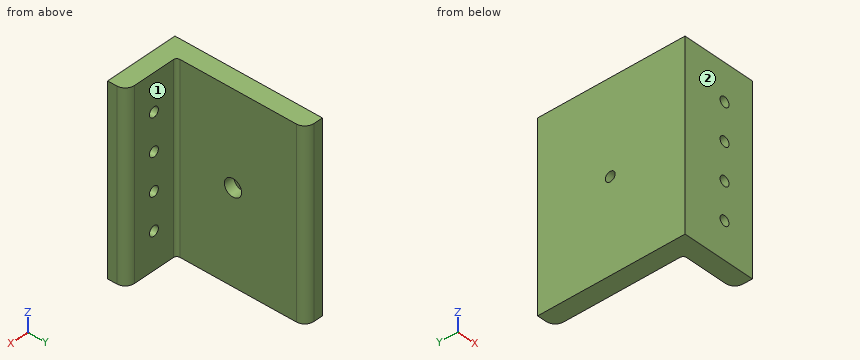
from build123d import *

# Parameters (mm, degrees)
L_ANGLE_L8X4X1_1_DEPTH                   = 254
F_1_2_CLEARANCE_HOLE1_D                  = 13.49248
CBORE_FOR_M12_HEX_HEAD_BOLT1_D           = 13.5
CBORE_FOR_M12_HEX_HEAD_BOLT1_CBORE_D     = 23.78
CBORE_FOR_M12_HEX_HEAD_BOLT1_CBORE_DEPTH = 14.3


with BuildPart() as part:
    # Sketch114 → L angle L8X4X1(1) (new body)
    with BuildSketch(Plane(origin=(390.937425431, -221.174980879, -159.063896304), x_dir=(1, 0, 0), z_dir=(0, 0, 1))):
        with BuildLine():
            Line((0, 0), (0, 203.2))
            Line((0, 203.2), (12.70508, 203.2))
            ThreePointArc((12.70508, 203.2), (21.681744019, 199.481744019), (25.4, 190.50508))
            Line((25.4, 190.50508), (25.4, 30.1625))
            ThreePointArc((25.4, 30.1625), (26.794903955, 26.794903955), (30.1625, 25.4))
            Line((30.1625, 25.4), (88.90508, 25.4))
            ThreePointArc((88.90508, 25.4), (97.881744019, 21.681744019), (101.6, 12.70508))
            Line((101.6, 12.70508), (101.6, 0))
            Line((101.6, 0), (0, 0))
        make_face()
    extrude(amount=L_ANGLE_L8X4X1_1_DEPTH)

    # 1/2 Clearance Hole1 (through all)
    with Locations(Plane(origin=(0, -195.774980879, 0), x_dir=(1, 0, 0), z_dir=(0, 1, 0))):
        with Locations((450.471215431, -44.136103696), (450.471215431, 108.263896304), (450.471215431, 57.463896304), (450.471215431, 6.663896304)):
            Hole(F_1_2_CLEARANCE_HOLE1_D / 2)

    # CBORE for M12 Hex Head Bolt1 (through all)
    with Locations(Plane(origin=(416.337425431, 0, 0), x_dir=(0, 0, -1), z_dir=(1, 0, 0))):
        with Locations((32.063896304, -118.000180879)):
            CounterBoreHole(CBORE_FOR_M12_HEX_HEAD_BOLT1_D / 2, CBORE_FOR_M12_HEX_HEAD_BOLT1_CBORE_D / 2, CBORE_FOR_M12_HEX_HEAD_BOLT1_CBORE_DEPTH)


solid = part.part
Geometry: final body of the model. Coordinates: model frame, mm. Face numbers are marked on the shaded views. A direction names the side the tool comes from. Coordinates: 2 decimals unless noted, no trailing zeros. Order: outer loops, then holes, each group sorted by start corner. A loop starts at its lowest first (then second) coordinate and runs counter-clockwise, first axis right, second up.
(1) First-contact query: pin 1 (12 mm diameter, centred on y = -118.5, z = -29, fed in from +X); pin 2 (8 mm diameter, centred on x = 478.5, z = -68, fed in from +Y) (3 decimals); pin 3 (12 mm diameter, centred on x = 450.47, z = -108.26, fed in from +Y); pin 4 (8 mm diameter, centred on y = -137, z = 38, fed in from +X). Flat tips, straight axial feed; report the tip coordinate or a pass-through.
(2) Section query D-D (z = 12). Return the cut outline in (x, y) (1 decimal).
(3) Section query C-C (y = -121.5). Return the cut outline in (x, z).
(4) Section query B-B (z = -32.5). Return the cut outline in (x, y) (1 decimal).
(5) Material intervals for probe 1 along Z at (x, y) = (414, -118); probe 2 along X at (y, z) = (-131, 40); probe 3 along Y at (x, z) = (471, -53), sorted ascending.
(6) Section query A-A (x = 452.5). Return the cut outline in (y, z), plus the area to 3 significant figures.
(7) Access query for the marked faces 1 and 2. Directions: +Z, -Z, +X, -X, +Y, -Y. A direction counts if a zero-diameter tool reaches every point of the face in a straight line with its end or side. Return the directions, or none.
Solution:
1. pin 1: stops at x = 402.04
1. pin 2: stops at y = -195.775
1. pin 3: passes through
1. pin 4: stops at x = 416.34
2. outline: (390.9, -221.2) - (492.5, -221.2) - (492.5, -208.5) arc R12.7 ccw to (479.8, -195.8) - (421.1, -195.8) arc R4.8 cw to (416.3, -191) - (416.3, -30.7) arc R12.7 ccw to (403.6, -18) - (390.9, -18) - close
3. outline: (390.94, -159.06) - (416.34, -159.06) - (416.34, -43.43) - (402.04, -43.43) - (402.04, -37.84) - (390.94, -37.84) - close; (390.94, -26.29) - (402.04, -26.29) - (402.04, -20.7) - (416.34, -20.7) - (416.34, 94.94) - (390.94, 94.94) - close
4. outline: (390.9, -221.2) - (492.5, -221.2) - (492.5, -208.5) arc R12.7 ccw to (479.8, -195.8) - (421.1, -195.8) arc R4.8 cw to (416.3, -191) - (416.3, -129.9) - (402, -129.9) - (402, -124.7) - (390.9, -124.7) - close; (390.9, -111.3) - (402, -111.3) - (402, -106.1) - (416.3, -106.1) - (416.3, -30.7) arc R12.7 ccw to (403.6, -18) - (390.9, -18) - close
5. probe 1: z = -159.06 to -43.95, -20.17 to 94.94
5. probe 2: x = 390.94 to 416.34
5. probe 3: y = -221.17 to -195.77
6. outline: (-221.17, -159.06) - (-195.77, -159.06) - (-195.77, -114.7) - (-221.17, -114.7) - close; (-221.17, -101.83) - (-195.77, -101.83) - (-195.77, -63.9) - (-221.17, -63.9) - close; (-221.17, -51.03) - (-195.77, -51.03) - (-195.77, -13.1) - (-221.17, -13.1) - close; (-221.17, -0.23) - (-195.77, -0.23) - (-195.77, 37.7) - (-221.17, 37.7) - close; (-221.17, 50.57) - (-195.77, 50.57) - (-195.77, 94.94) - (-221.17, 94.94) - close
6. area: 5,140 mm2
7. face 1: +Z, -Z, +X, +Y
7. face 2: +Z, -Z, +X, -X, -Y
